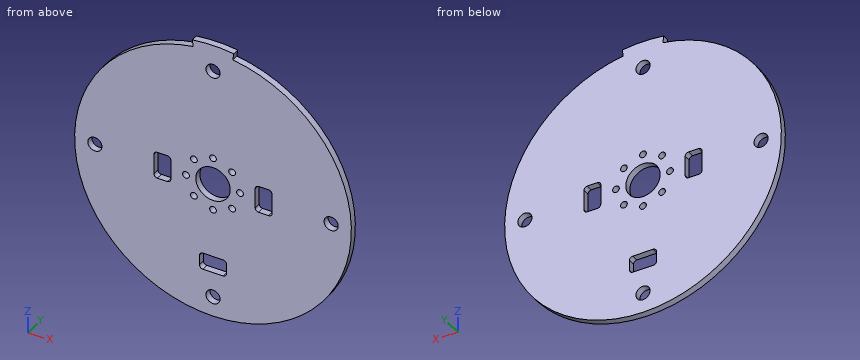
```python
from build123d import *

# Parameters (mm, degrees)
SM_BASE_FLANGE_1_DEPTH = 2
CUT_EXTRUDE_1_REACH    = 61.447
SKETCH_6_R             = 2.1
SKETCH_6_R_2           = 5.1
SKETCH_6_R_3           = 1
SKETCH_6_W             = 8
SKETCH_6_H             = 5
SKETCH_6_W_2           = 5
SKETCH_6_H_2           = 8
FILLET_1_R             = 1


# Sheet-metal steps are written as plain solids
with BuildPart() as part:
    # Sketch 1 → 基体-法兰1 (new body)
    with BuildSketch(Plane(origin=(0, 0, 0), x_dir=(1, 0, 0), z_dir=(0, 1, 0))):
        with BuildLine():
            Line((-6.14057756, -42.559291667), (-5.854969301, -40.579789729))
            ThreePointArc((-5.854969301, -40.579789729), (-0.00413932, 40.999999791), (5.863162974, -40.578606678))
            Line((5.863162974, -40.578606678), (6.149170924, -42.558050906))
            ThreePointArc((6.149170924, -42.558050906), (0.004341238, -42.999999781), (-6.14057756, -42.559291667))
        make_face()
    extrude(amount=-SM_BASE_FLANGE_1_DEPTH)

    # 草图6 → 切除-拉伸1 (cut, up to next)
    with BuildSketch(Plane(origin=(0, 0, 0), x_dir=(1, 0, 0), z_dir=(0, 1, 0)), mode=Mode.PRIVATE) as cut_extrude_1_sk1:
        with Locations(Location((0, 35, 0), (0, 0, 270))):
            Circle(SKETCH_6_R)
    cut_extrude_1_tool1 = extrude(cut_extrude_1_sk1.sketch, amount=-CUT_EXTRUDE_1_REACH, mode=Mode.PRIVATE) & part.part
    # 草图6 → 切除-拉伸1 (cut, up to next)
    with BuildSketch(Plane(origin=(0, 0, 0), x_dir=(1, 0, 0), z_dir=(0, 1, 0)), mode=Mode.PRIVATE) as cut_extrude_1_sk2:
        with Locations(Location((35, 0, 0), (0, 0, 270))):
            Circle(SKETCH_6_R)
    cut_extrude_1_tool2 = extrude(cut_extrude_1_sk2.sketch, amount=-CUT_EXTRUDE_1_REACH, mode=Mode.PRIVATE) & part.part
    # 草图6 → 切除-拉伸1 (cut, up to next)
    with BuildSketch(Plane(origin=(0, 0, 0), x_dir=(1, 0, 0), z_dir=(0, 1, 0)), mode=Mode.PRIVATE) as cut_extrude_1_sk3:
        with Locations(Location((0, -35, 0), (0, 0, 270))):
            Circle(SKETCH_6_R)
    cut_extrude_1_tool3 = extrude(cut_extrude_1_sk3.sketch, amount=-CUT_EXTRUDE_1_REACH, mode=Mode.PRIVATE) & part.part
    # 草图6 → 切除-拉伸1 (cut, up to next)
    with BuildSketch(Plane(origin=(0, 0, 0), x_dir=(1, 0, 0), z_dir=(0, 1, 0)), mode=Mode.PRIVATE) as cut_extrude_1_sk4:
        with Locations(Location((-35, 0, 0), (0, 0, 270))):
            Circle(SKETCH_6_R)
    cut_extrude_1_tool4 = extrude(cut_extrude_1_sk4.sketch, amount=-CUT_EXTRUDE_1_REACH, mode=Mode.PRIVATE) & part.part
    # 草图6 → 切除-拉伸1 (cut, up to next)
    with BuildSketch(Plane(origin=(0, 0, 0), x_dir=(1, 0, 0), z_dir=(0, 1, 0)), mode=Mode.PRIVATE) as cut_extrude_1_sk5:
        with Locations(Location((0, 0, 0), (0, 0, 270))):
            Circle(SKETCH_6_R_2)
    cut_extrude_1_tool5 = extrude(cut_extrude_1_sk5.sketch, amount=-CUT_EXTRUDE_1_REACH, mode=Mode.PRIVATE) & part.part
    # 草图6 → 切除-拉伸1 (cut, up to next)
    with BuildSketch(Plane(origin=(0, 0, 0), x_dir=(1, 0, 0), z_dir=(0, 1, 0)), mode=Mode.PRIVATE) as cut_extrude_1_sk6:
        with Locations(Location((0, 8, 0), (0, 0, 270))):
            Circle(SKETCH_6_R_3)
    cut_extrude_1_tool6 = extrude(cut_extrude_1_sk6.sketch, amount=-CUT_EXTRUDE_1_REACH, mode=Mode.PRIVATE) & part.part
    # 草图6 → 切除-拉伸1 (cut, up to next)
    with BuildSketch(Plane(origin=(0, 0, 0), x_dir=(1, 0, 0), z_dir=(0, 1, 0)), mode=Mode.PRIVATE) as cut_extrude_1_sk7:
        with Locations(Location((5.656854249, 5.656854249, 0), (0, 0, 270))):
            Circle(SKETCH_6_R_3)
    cut_extrude_1_tool7 = extrude(cut_extrude_1_sk7.sketch, amount=-CUT_EXTRUDE_1_REACH, mode=Mode.PRIVATE) & part.part
    # 草图6 → 切除-拉伸1 (cut, up to next)
    with BuildSketch(Plane(origin=(0, 0, 0), x_dir=(1, 0, 0), z_dir=(0, 1, 0)), mode=Mode.PRIVATE) as cut_extrude_1_sk8:
        with Locations(Location((8, 0, 0), (0, 0, 270))):
            Circle(SKETCH_6_R_3)
    cut_extrude_1_tool8 = extrude(cut_extrude_1_sk8.sketch, amount=-CUT_EXTRUDE_1_REACH, mode=Mode.PRIVATE) & part.part
    # 草图6 → 切除-拉伸1 (cut, up to next)
    with BuildSketch(Plane(origin=(0, 0, 0), x_dir=(1, 0, 0), z_dir=(0, 1, 0)), mode=Mode.PRIVATE) as cut_extrude_1_sk9:
        with Locations(Location((5.656854249, -5.656854249, 0), (0, 0, 270))):
            Circle(SKETCH_6_R_3)
    cut_extrude_1_tool9 = extrude(cut_extrude_1_sk9.sketch, amount=-CUT_EXTRUDE_1_REACH, mode=Mode.PRIVATE) & part.part
    # 草图6 → 切除-拉伸1 (cut, up to next)
    with BuildSketch(Plane(origin=(0, 0, 0), x_dir=(1, 0, 0), z_dir=(0, 1, 0)), mode=Mode.PRIVATE) as cut_extrude_1_sk10:
        with Locations(Location((0, -8, 0), (0, 0, 270))):
            Circle(SKETCH_6_R_3)
    cut_extrude_1_tool10 = extrude(cut_extrude_1_sk10.sketch, amount=-CUT_EXTRUDE_1_REACH, mode=Mode.PRIVATE) & part.part
    # 草图6 → 切除-拉伸1 (cut, up to next)
    with BuildSketch(Plane(origin=(0, 0, 0), x_dir=(1, 0, 0), z_dir=(0, 1, 0)), mode=Mode.PRIVATE) as cut_extrude_1_sk11:
        with Locations(Location((-5.656854249, -5.656854249, 0), (0, 0, 270))):
            Circle(SKETCH_6_R_3)
    cut_extrude_1_tool11 = extrude(cut_extrude_1_sk11.sketch, amount=-CUT_EXTRUDE_1_REACH, mode=Mode.PRIVATE) & part.part
    # 草图6 → 切除-拉伸1 (cut, up to next)
    with BuildSketch(Plane(origin=(0, 0, 0), x_dir=(1, 0, 0), z_dir=(0, 1, 0)), mode=Mode.PRIVATE) as cut_extrude_1_sk12:
        with Locations(Location((-8, 0, 0), (0, 0, 270))):
            Circle(SKETCH_6_R_3)
    cut_extrude_1_tool12 = extrude(cut_extrude_1_sk12.sketch, amount=-CUT_EXTRUDE_1_REACH, mode=Mode.PRIVATE) & part.part
    # 草图6 → 切除-拉伸1 (cut, up to next)
    with BuildSketch(Plane(origin=(0, 0, 0), x_dir=(1, 0, 0), z_dir=(0, 1, 0)), mode=Mode.PRIVATE) as cut_extrude_1_sk13:
        with Locations(Location((-5.656854249, 5.656854249, 0), (0, 0, 270))):
            Circle(SKETCH_6_R_3)
    cut_extrude_1_tool13 = extrude(cut_extrude_1_sk13.sketch, amount=-CUT_EXTRUDE_1_REACH, mode=Mode.PRIVATE) & part.part
    # 草图6 → 切除-拉伸1 (cut, up to next)
    with BuildSketch(Plane(origin=(0, 0, 0), x_dir=(1, 0, 0), z_dir=(0, 1, 0)), mode=Mode.PRIVATE) as cut_extrude_1_sk14:
        with Locations((0, 25)):
            Rectangle(SKETCH_6_W, SKETCH_6_H)
    cut_extrude_1_tool14 = extrude(cut_extrude_1_sk14.sketch, amount=-CUT_EXTRUDE_1_REACH, mode=Mode.PRIVATE) & part.part
    # 草图6 → 切除-拉伸1 (cut, up to next)
    with BuildSketch(Plane(origin=(0, 0, 0), x_dir=(1, 0, 0), z_dir=(0, 1, 0)), mode=Mode.PRIVATE) as cut_extrude_1_sk15:
        with Locations((15, 0)):
            Rectangle(SKETCH_6_W_2, SKETCH_6_H_2)
    cut_extrude_1_tool15 = extrude(cut_extrude_1_sk15.sketch, amount=-CUT_EXTRUDE_1_REACH, mode=Mode.PRIVATE) & part.part
    # 草图6 → 切除-拉伸1 (cut, up to next)
    with BuildSketch(Plane(origin=(0, 0, 0), x_dir=(1, 0, 0), z_dir=(0, 1, 0)), mode=Mode.PRIVATE) as cut_extrude_1_sk16:
        with Locations((-15, 0)):
            Rectangle(SKETCH_6_W_2, SKETCH_6_H_2)
    cut_extrude_1_tool16 = extrude(cut_extrude_1_sk16.sketch, amount=-CUT_EXTRUDE_1_REACH, mode=Mode.PRIVATE) & part.part
    add(cut_extrude_1_tool1.solids().sort_by_distance((0, 0, -35))[0], mode=Mode.SUBTRACT)
    add(cut_extrude_1_tool2.solids().sort_by_distance((35, 0, 0))[0], mode=Mode.SUBTRACT)
    add(cut_extrude_1_tool3.solids().sort_by_distance((0, 0, 35))[0], mode=Mode.SUBTRACT)
    add(cut_extrude_1_tool4.solids().sort_by_distance((-35, 0, 0))[0], mode=Mode.SUBTRACT)
    add(cut_extrude_1_tool5.solids().sort_by_distance((0, 0, 0))[0], mode=Mode.SUBTRACT)
    add(cut_extrude_1_tool6.solids().sort_by_distance((0, 0, -8))[0], mode=Mode.SUBTRACT)
    add(cut_extrude_1_tool7.solids().sort_by_distance((5.656854, 0, -5.656854))[0], mode=Mode.SUBTRACT)
    add(cut_extrude_1_tool8.solids().sort_by_distance((8, 0, 0))[0], mode=Mode.SUBTRACT)
    add(cut_extrude_1_tool9.solids().sort_by_distance((5.656854, 0, 5.656854))[0], mode=Mode.SUBTRACT)
    add(cut_extrude_1_tool10.solids().sort_by_distance((0, 0, 8))[0], mode=Mode.SUBTRACT)
    add(cut_extrude_1_tool11.solids().sort_by_distance((-5.656854, 0, 5.656854))[0], mode=Mode.SUBTRACT)
    add(cut_extrude_1_tool12.solids().sort_by_distance((-8, 0, 0))[0], mode=Mode.SUBTRACT)
    add(cut_extrude_1_tool13.solids().sort_by_distance((-5.656854, 0, -5.656854))[0], mode=Mode.SUBTRACT)
    add(cut_extrude_1_tool14.solids().sort_by_distance((0, 0, -25))[0], mode=Mode.SUBTRACT)
    add(cut_extrude_1_tool15.solids().sort_by_distance((15, 0, 0))[0], mode=Mode.SUBTRACT)
    add(cut_extrude_1_tool16.solids().sort_by_distance((-15, 0, 0))[0], mode=Mode.SUBTRACT)

    # 圆角1
    fillet_1_edges = [part.edges().sort_by_distance(p)[0] for p in [
        (-17.5, -1, 4),
        (-17.5, -1, -4),
        (-12.5, -1, -4),
        (-12.5, -1, 4),
        (12.5, -1, 4),
        (12.5, -1, -4),
        (17.5, -1, -4),
        (17.5, -1, 4),
        (-4, -1, -22.5),
        (-4, -1, -27.5),
        (4, -1, -27.5),
        (4, -1, -22.5),
    ]]
    fillet(fillet_1_edges, radius=FILLET_1_R)


solid = part.part
```
The model under review builds one solid part; all positions refer to its coordinate system, in mm. Give positions to 0.01 mm unless a question says otherwise; leave off trailing zeros. Write each loop counter-clockwise with the first axis right and the second up, starting at its lowest first coordinate (ties: lowest second). Pieces come first, ordered by that corner, then holes. Notation, with made-up numbers: (84, -17.75) -> (121, -17.75) arc R17 cw to (121, 3.25) -> close; hole circle Ø9 at (-12, -10.75). An arc over 180 degrees is marked (long way). Put each result on its own line as item: value.
(1) We need section B-B, the plane x = 8. Give the boundary of the cut face in (y, z).
Results are:
outline: (-2, -40.21) -> (0, -40.21) -> (0, -1) -> (-2, -1) -> close; (-2, 1) -> (0, 1) -> (0, 40.21) -> (-2, 40.21) -> close
(2) To check wall thickness, follow probe 1 along Z at (x, y) = (-3, -1.7); probe 2 along Z at (x, y) = (-3.5, -1.15); probe 3 along Z at (x, y) = (13, -1.5). State the ranges of each line that lie inside material, in increasing order. Write a range as from..to.
Results are:
probe 1: -40.89..-27.5, -22.5..-4.12, 4.12..42.9
probe 2: -40.85..-27.37, -22.63..-3.71, 3.71..42.86
probe 3: -38.88..-3.87, 3.87..38.88
(3) We need section A-A, the plane z = 0. State how many separate pieces and enclosed holes the cut face has, and give its area (3 significant figures).
Results are:
separate pieces: 8
enclosed holes: 0
area: 98.8 mm²
(4) We need section C-C, the plane z = 35. Give the boundary of the cut face in (x, y), and give its area (3 significant figures).
Results are:
outline: (-21.35, -2) -> (-2.1, -2) -> (-2.1, 0) -> (-21.35, 0) -> close; (2.1, -2) -> (21.35, -2) -> (21.35, 0) -> (2.1, 0) -> close
area: 77.0 mm²
(5) For pin 1 Ø1 at (x, y) = (22, -1) entering from +Z; pin 2 Ø6.5 at (x, z) = (0, 35) entering from -Y; pin 3 Ø1.6 at (x, z) = (-5.66, -5.66) entering from +Y; pin 4 Ø0.6 at (y, z) = (-1.5, -25) entering from +X, all flat-tipped, find the tip position at first contact; note any pin that passes through.
Results are:
pin 1: z = 34.91
pin 2: y = -2
pin 3: through
pin 4: x = 32.72
